```python
from build123d import *

# Parameters (mm, degrees)
F0_R     = 31.75
F1_DEPTH = 1.27
F2_R     = 19.05
F3_DEPTH = 12.7
F4_R     = 31.75
F5_DEPTH = 1.27
F7_D     = 20.32
F8_D     = 20.32
F9_D     = 20.32
F11_D    = 15.24


with BuildPart() as f1:
    # F0 (on Top) → F1 (new body)
    with BuildSketch(Plane.XY):
        Circle(F0_R)
    extrude(amount=F1_DEPTH)

    # F2 (on face) → F3 (join)
    with BuildSketch(Plane.XY.offset(1.27)):
        Circle(F2_R)
    extrude(amount=F3_DEPTH)

    # F4 (on face) → F5 (join)
    with BuildSketch(Plane.XY.offset(13.97)):
        Circle(F4_R)
    extrude(amount=F5_DEPTH)

    # F7 (through all)
    with Locations(Plane.XY.offset(15.24)):
        with Locations((17.50788, 9.938807)):
            Hole(F7_D / 2)

    # F8 (through all)
    with Locations(Plane.XY.offset(15.24)):
        with Locations((-0.146656, -20.12828)):
            Hole(F8_D / 2)

    # F9 (through all)
    with Locations(Plane.XY.offset(15.24)):
        with Locations((-17.359468, 10.191849)):
            Hole(F9_D / 2)

    # F11 (through all)
    with Locations(Plane.XY.offset(15.24)):
        with Locations((0, 0)):
            Hole(F11_D / 2)


solid = f1.part
```
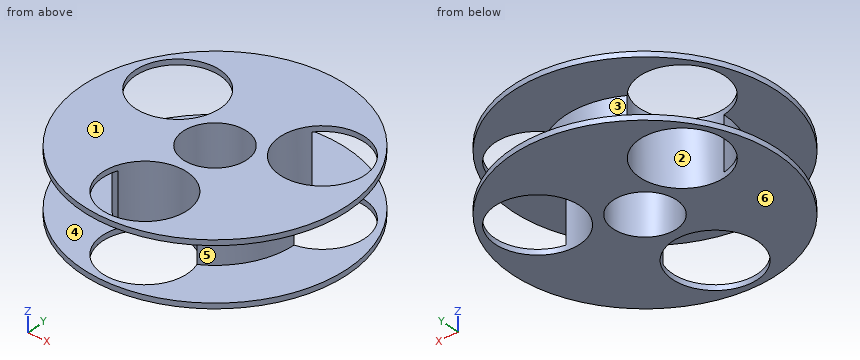
Geometry: final body of the model. Coordinates: model frame, mm. Face numbers are marked on the shaded views. A direction names the side the tool comes from. Give positions to 0.01 mm unless a question says otherwise; leave off trailing zeros. Order: outer loops, then holes, each group sorted by start corner. A loop starts at its lowest first (then second) coordinate and runs counter-clockwise, first axis right, second up. Notation, with made-up numbers: (42.5, 33) -> (49.5, 33) arc R20 cw to (49.5, 61) -> close; hole circle Ø3 at (-6, 66). An arc over 180 degrees is marked (long way). Write each question's results on one line, items separated by ' | '. Start each with the question number.
1) Section A-A (y = -21). Return loops of the section in (x, z), then the cut area to 3 significant figures.
2) Section C-C (y = -11). Return loops of the section in (x, z), then the cut area to 3 significant figures.
3) Line query: line 1 (Y direction, x = 0, z = 11); line 2 (Z direction, x = 21.5, y = -5); line 3 (X direction, y = 4.5, z = 14). Output: solid intervals per line, ascending. Write a range as from..to.
4) Section B-B (x = 0). Return loops of the section in (y, z), then the cut area to 3 significant figures.
5) Section D-D (z = 8). Return loops of the section in (x, y), then the cut area to 3 significant figures.
6) Draft query along X for the marked faces 1, 2 and 3. Return one class per face: pulls with the +X half, pulls with the -X half, needs draft (parallel to the pull), parting line crosses it, or undercut.
7) Set-up query: the marked faces 4, 5 and 6. Return all of +Z, -Z, +X, -X, +Y, -Y with unobstructed straight access to the full face (end or side cutting, diameter ignored); none if empty.
8) First-contact query: pin 1 (8 mm diameter, centred on y = -22, z = 5, fed in from +X); pin 2 (6 mm diameter, centred on x = 13, z = 12, fed in from +Y); pin 3 (17.5 mm diameter, centred on x = 0, y = 0, fed in from -Z); pin 4 (4 mm diameter, centred on x = -3.5, z = 7, fed in from -Y). Flat tips, straight axial feed; report the tip coordinate or a pass-through.
Calculated:
1) outline: (-23.81, 0) -> (-10.27, 0) -> (-10.27, 1.27) -> (-23.81, 1.27) -> close; (-23.81, 13.97) -> (-10.27, 13.97) -> (-10.27, 15.24) -> (-23.81, 15.24) -> close; (9.98, 0) -> (23.81, 0) -> (23.81, 1.27) -> (9.98, 1.27) -> close; (9.98, 13.97) -> (23.81, 13.97) -> (23.81, 15.24) -> (9.98, 15.24) -> close | area: 69.5 mm2
2) outline: (-29.78, 0) -> (-4.61, 0) -> (-4.61, 15.24) -> (-29.78, 15.24) -> (-29.78, 13.97) -> (-15.55, 13.97) -> (-15.55, 1.27) -> (-29.78, 1.27) -> close; (4.31, 0) -> (29.78, 0) -> (29.78, 1.27) -> (15.55, 1.27) -> (15.55, 13.97) -> (29.78, 13.97) -> (29.78, 15.24) -> (4.31, 15.24) -> close | area: 410 mm2
3) line 1: -9.97..-7.62, 7.62..19.05 | line 2: 0..1.27, 13.97..15.24 | line 3: -31.43..-25.78, -8.94..-6.15, 6.15..8.93, 26.09..31.43
4) outline: (-31.75, 0) -> (-30.29, 0) -> (-30.29, 1.27) -> (-31.75, 1.27) -> close; (-31.75, 13.97) -> (-30.29, 13.97) -> (-30.29, 15.24) -> (-31.75, 15.24) -> close; (-9.97, 0) -> (-7.62, 0) -> (-7.62, 15.24) -> (-9.97, 15.24) -> close; (7.62, 0) -> (31.75, 0) -> (31.75, 1.27) -> (19.05, 1.27) -> (19.05, 13.97) -> (31.75, 13.97) -> (31.75, 15.24) -> (7.62, 15.24) -> close | area: 246 mm2
5) outline: (-19.05, 0.17) arc R19.05 ccw to (-9.62, -16.45) arc R10.16 cw to (9.37, -16.58) arc R19.05 ccw to (19.05, -0.1) arc R10.16 cw to (9.68, 16.41) arc R19.05 ccw to (-9.43, 16.55) arc R10.16 cw to start; hole circle Ø15.24 at (0, 0) | area: 589 mm2
6) face 1: needs draft | face 2: undercut | face 3: parting line crosses it
7) face 4: none | face 5: +X, -Y | face 6: -Z, +X, -X, +Y, -Y
8) pin 1: x = 24.2 | pin 2: y = 29.88 | pin 3: z = 0 | pin 4: y = -11.49
